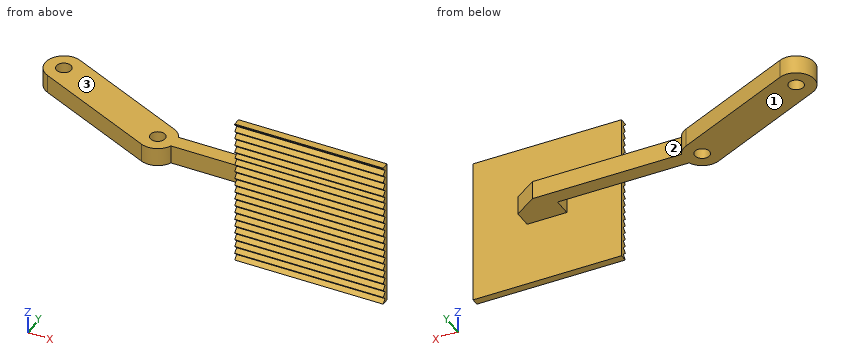
from build123d import *

# Parameters (mm, degrees)
SKETCH_1_R          = 2
EXTRUDE_1_DEPTH     = 2.5
SKETCH_2_W          = 40
SKETCH_2_H          = 40
EXTRUDE_2_DEPTH     = 2
CUT_EXTRUDE_1_DEPTH = 40


with BuildPart() as part:
    # 草图1 → 凸台-拉伸1 (new, symmetric)
    with BuildSketch(Plane.XY):
        with BuildLine():
            Line((2.069014722, 4.551832387), (35.069014722, -10.448167613))
            ThreePointArc((35.069014722, -10.448167613), (36.562144846, -11.491278851), (37.582575695, -13))
            Line((37.582575695, -13), (73, -13))
            Line((73, -13), (77.669363216, -13))
            Line((77.669363216, -13), (83.69352751, -17))
            Line((83.69352751, -17), (83.69352751, -21.856832822))
            Line((83.69352751, -21.856832822), (73, -21.856832822))
            Line((73, -21.856832822), (73, -17))
            Line((73, -17), (37.582575695, -17))
            ThreePointArc((37.582575695, -17), (34.790938113, -19.668248138), (30.930985278, -19.551832387))
            Line((30.930985278, -19.551832387), (-2.069014722, -4.551832387))
            ThreePointArc((-2.069014722, -4.551832387), (-4.551832387, 2.069014722), (2.069014722, 4.551832387))
        make_face()
        Circle(SKETCH_1_R, mode=Mode.SUBTRACT)
        with Locations((33, -15)):
            Circle(SKETCH_1_R, mode=Mode.SUBTRACT)
    extrude(amount=EXTRUDE_1_DEPTH, both=True)

    # 草图2 → 凸台-拉伸2 (add)
    with BuildSketch(Plane.XZ.offset(21.856832822)):
        with Locations((78.275712014, 0)):
            Rectangle(SKETCH_2_W, SKETCH_2_H)
    extrude(amount=EXTRUDE_2_DEPTH)

    # 草图4 → 切除-拉伸1 (cut)
    with BuildSketch(Plane.ZY.offset(-58.275712014)):
        Polygon((-19, -22.856832822), (-20, -23.856832822), (-18, -23.856832822), align=None)
        Polygon((-17, -22.856832822), (-18, -23.856832822), (-16, -23.856832822), align=None)
        Polygon((-15, -22.856832822), (-16, -23.856832822), (-14, -23.856832822), align=None)
        Polygon((-13, -22.856832822), (-14, -23.856832822), (-12, -23.856832822), align=None)
        Polygon((-11, -22.856832822), (-12, -23.856832822), (-10, -23.856832822), align=None)
        Polygon((-9, -22.856832822), (-10, -23.856832822), (-8, -23.856832822), align=None)
        Polygon((-7, -22.856832822), (-8, -23.856832822), (-6, -23.856832822), align=None)
        Polygon((-5, -22.856832822), (-6, -23.856832822), (-4, -23.856832822), align=None)
        Polygon((-3, -22.856832822), (-4, -23.856832822), (-2, -23.856832822), align=None)
        Polygon((-1, -22.856832822), (-2, -23.856832822), (0, -23.856832822), align=None)
        Polygon((1, -22.856832822), (0, -23.856832822), (2, -23.856832822), align=None)
        Polygon((3, -22.856832822), (2, -23.856832822), (4, -23.856832822), align=None)
        Polygon((5, -22.856832822), (4, -23.856832822), (6, -23.856832822), align=None)
        Polygon((7, -22.856832822), (6, -23.856832822), (8, -23.856832822), align=None)
        Polygon((9, -22.856832822), (8, -23.856832822), (11.695910697, -23.856832822), (10.695910697, -22.856832822), (9.847955349, -23.70478817), align=None)
        Polygon((12.695910697, -22.856832822), (11.695910697, -23.856832822), (13.695910697, -23.856832822), align=None)
        Polygon((18.695910697, -22.856832822), (17.695910697, -23.856832822), (19.695910697, -23.856832822), align=None)
        Polygon((16.695910697, -22.856832822), (15.695910697, -23.856832822), (17.695910697, -23.856832822), align=None)
        Polygon((14.695910697, -22.856832822), (13.695910697, -23.856832822), (15.695910697, -23.856832822), align=None)
    extrude(amount=-CUT_EXTRUDE_1_DEPTH, mode=Mode.SUBTRACT)


solid = part.part
Input: part model. Units: mm. Frame: model coordinates. Face numbers are marked on the shaded views. A direction names the side the tool comes from. Give positions to 0.01 mm unless a question says otherwise; leave off trailing zeros. Write each loop counter-clockwise with the first axis right and the second up, starting at its lowest first coordinate (ties: lowest second). Pieces come first, ordered by that corner, then holes.
Q1. Section C-C, the plane y = -9. Output: boundary loops of the cut face in (x, z), plus the area to 3 significant figures.
Q2. First-contact query: P1, Ø5, axis at x = 80, z = -15, coming from the +Y side; P2, Ø1.5, axis at x = 47, z = -1, coming from the -Y side; P3, Ø10, axis at y = -7.5, z = -6, coming from the -X side; P4, Ø1, axis at x = 85, y = -20.5, coming from the +Z side. Flat tips, straight axial feed; report the tip coordinate or a pass-through.
Q3. Set-up query: the marked faces 1, 2 and 3. Return all of +Z, -Z, +X, -X, +Y, -Y with unobstructed straight access to the full face (end or side cutting, diameter ignored); none if empty.
Q4. Section A-A, the plane y = 0. Output: boundary loops of the cut face in (x, z).
Q5. Material intervals for probe 1 along Z at (x, y) = (25.5, -11); probe 2 along Y at (x, z) = (0, -0.9); probe 3 along Y at (x, z) = (33, 0.3), sorted ascending.
Q6. Section D-D, the plane x = 22. Output: boundary loops of the cut face in (y, z).
Q7. Section B-B, the plane x = 0. Output: boundary loops of the cut face in (y, z), plus the area to 3 significant figures.
Filled in:
1. outline: (7.72, -2.5) - (31.88, -2.5) - (31.88, 2.5) - (7.72, 2.5) - close
1. area: 121 mm2
2. P1: stops at y = -21.86
2. P2: stops at y = -17
2. P3: stops at x = -3.09
2. P4: passes through
3. face 1: -Z, +X, -X, +Y
3. face 2: +Z, -Z, +X, +Y
3. face 3: +Z, +X, -X, +Y
4. outline: (-5, -2.5) - (-2, -2.5) - (-2, 2.5) - (-5, 2.5) - close; (2, -2.5) - (12.08, -2.5) - (12.08, 2.5) - (2, 2.5) - close
5. probe 1: z = -2.5 to 2.5
5. probe 2: y = -5.49 to -2, 2 to 5
5. probe 3: y = -20 to -17, -13 to -9.51
6. outline: (-15.49, -2.5) - (-4.51, -2.5) - (-4.51, 2.5) - (-15.49, 2.5) - close
7. outline: (-5.49, -2.5) - (-2, -2.5) - (-2, 2.5) - (-5.49, 2.5) - close; (2, -2.5) - (5, -2.5) - (5, 2.5) - (2, 2.5) - close
7. area: 32.5 mm2
